from build123d import *

# Parameters (mm, degrees)
SKETCH1_W           = 60
SKETCH1_H           = 165
BOSS_EXTRUDE1_DEPTH = 5
SKETCH2_W           = 50
SKETCH2_H           = 50
BOSS_EXTRUDE3_DEPTH = 2
LPATTERN1_COUNT     = 3
LPATTERN1_PITCH     = 52
SKETCH3_W           = 52
SKETCH3_H           = 51.9
BOSS_EXTRUDE8_DEPTH = 25
LPATTERN5_COUNT     = 3
LPATTERN5_PITCH     = 52


with BuildPart() as part:
    # Sketch1 → Boss-Extrude1 (new body)
    with BuildSketch(Plane(origin=(0, 0, 0), x_dir=(1, 0, 0), z_dir=(0, 1, 0))):
        Rectangle(SKETCH1_W, SKETCH1_H)
    extrude(amount=BOSS_EXTRUDE1_DEPTH)

    # Sketch2 → Boss-Extrude3 (add)
    with BuildSketch(Plane(origin=(0, 5, 0), x_dir=(1, 0, 0), z_dir=(0, 1, 0))):
        with Locations((0, -52.5)):
            Rectangle(SKETCH2_W, SKETCH2_H)
    boss_extrude3 = extrude(amount=BOSS_EXTRUDE3_DEPTH)

    # LPattern1: Boss-Extrude3 ×3
    with Locations(*[(0, 0, -i * LPATTERN1_PITCH) for i in range(1, LPATTERN1_COUNT)]):
        add(boss_extrude3)

    # Sketch3 → Boss-Extrude8 (add)
    with BuildSketch(Plane(origin=(0, 7, 0), x_dir=(1, 0, 0), z_dir=(0, 1, 0))):
        with Locations((0, -52.55)):
            Rectangle(SKETCH3_W, SKETCH3_H)
    boss_extrude8 = extrude(amount=BOSS_EXTRUDE8_DEPTH)

    # LPattern5: Boss-Extrude8 ×3
    with Locations(*[(0, 0, -i * LPATTERN5_PITCH) for i in range(1, LPATTERN5_COUNT)]):
        add(boss_extrude8)


solid = part.part
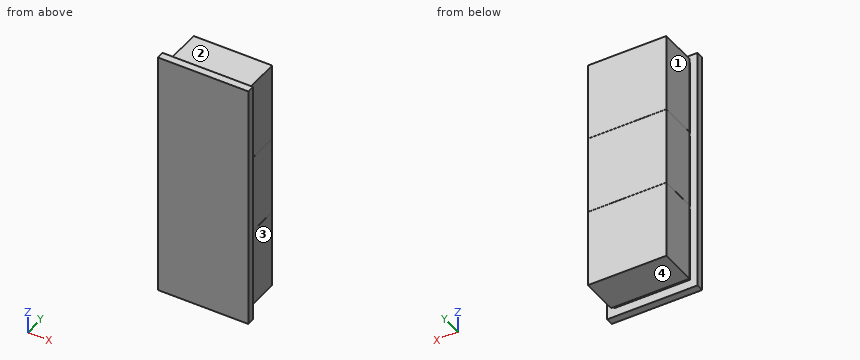
The model under review builds one solid part; all positions refer to its coordinate system, in mm. Face numbers are marked on the shaded views. A direction names the side the tool comes from. Give positions to 0.01 mm unless a question says otherwise; leave off trailing zeros. Loops run counter-clockwise (first coordinate to the right, second up) from the corner with the lowest first, then second, coordinate; pieces in that order, holes last. Notation, with made-up numbers: (84, 41.5) -> (143, 41.5) arc R18 ccw to (143, 72.5) -> close; hole circle Ø5 at (55, -33). An arc over 180 degrees is marked (long way). Answer as a JSON object with one key per item and string values. Group by question number.
Q1. Take a section at B-B (z = 10.5). Write out the cut boundary in (x, y).
Q2. Wall thickness on line 1 along X through (y, z) = (16.5, 44.5): over which ranges is the line inside the solid? List them lowest first.
Q3. Take a section at A-A (y = 22). Write out the cut boundary in (x, z).
Q4. Take a section at C-C (x = 1). Write out the cut boundary in (y, z), plus the area to 3 significant figures.
Q5. Tool access review of the marked faces 1, 2, 3 and 4: name each direction out of +Z, -Z, +X, -X, +Y, -Y from which nothing blocks a thin tool from reaching the whole face with its end or side.
Q6. Insertion check: pin 1 (0.6 mm diameter, centred on x = 4, y = 6, fed in from -Z); pin 2 (1 mm diameter, centred on x = 11.5, y = 6, fed in from +Z); pin 3 (0.6 mm diameter, centred on y = 5.5, z = -58, fed in from -X); pin 4 (10 mm diameter, centred on x = 13.5, z = 23, fed in from -Y). Each pin has a flat end and moves straight along its axis. Give the tip position at first contact, or say it passes through.
Answer below:
{
 "1": {"outline": "(-30, 0) -> (30, 0) -> (30, 5) -> (25, 5) -> (25, 7) -> (26, 7) -> (26, 32) -> (-26, 32) -> (-26, 7) -> (-25, 7) -> (-25, 5) -> (-30, 5) -> close"},
 "2": {"line 1": "x = -26 to 26"},
 "3": {"outline": "(-26, -77.4) -> (26, -77.4) -> (26, -25.5) -> (-26, -25.5) -> close; (-26, -25.4) -> (26, -25.4) -> (26, 26.5) -> (-26, 26.5) -> close; (-26, 26.6) -> (26, 26.6) -> (26, 78.5) -> (-26, 78.5) -> close"},
 "4": {"outline": "(0, -82.5) -> (5, -82.5) -> (5, -76.5) -> (7, -76.5) -> (7, -77.4) -> (32, -77.4) -> (32, -25.5) -> (7, -25.5) -> (7, -26.5) -> (5, -26.5) -> (5, -24.5) -> (7, -24.5) -> (7, -25.4) -> (32, -25.4) -> (32, 26.5) -> (7, 26.5) -> (7, 25.5) -> (5, 25.5) -> (5, 27.5) -> (7, 27.5) -> (7, 26.6) -> (32, 26.6) -> (32, 78.5) -> (7, 78.5) -> (7, 77.5) -> (5, 77.5) -> (5, 82.5) -> (0, 82.5) -> close", "area": "5,020 mm2"},
 "5": {"face 1": "+Z, -Z, -X, +Y", "face 2": "+Z, +X, -X, +Y", "face 3": "+Z, -Z, +X, +Y", "face 4": "-Z, +X, -X, +Y"},
 "6": {"pin 1": "stops at z = -76.5", "pin 2": "stops at z = 77.5", "pin 3": "stops at x = -25", "pin 4": "stops at y = 0"}
}
